```python
from build123d import *

# Parameters (mm, degrees)
SKETCH1_R           = 11.1125
BOSS_EXTRUDE1_DEPTH = 23.8125


with BuildPart() as part:
    # Sketch1 → Boss-Extrude1 (new body)
    with BuildSketch(Plane.XY):
        with BuildLine():
            Line((-19.45060256, -8.998474127), (-11.749724448, -25.644265115))
            Line((-11.749724448, -25.644265115), (12.863242985, -25.644265115))
            Line((12.863242985, -25.644265115), (19.45060256, -8.998474127))
            ThreePointArc((19.45060256, -8.998474127), (21.400108774, 1.154911696), (18.369201048, 11.039516721))
            Line((18.369201048, 11.039516721), (31.970540917, 23.950858732))
            Line((31.970540917, 23.950858732), (25.535140583, 31.951663088))
            Line((25.535140583, 31.951663088), (11.153892049, 18.299977287))
            ThreePointArc((11.153892049, 18.299977287), (-14.265700604, 15.993381845), (-19.45060256, -8.998474127))
        make_face()
        Circle(SKETCH1_R, mode=Mode.SUBTRACT)
    extrude(amount=BOSS_EXTRUDE1_DEPTH)


solid = part.part
```
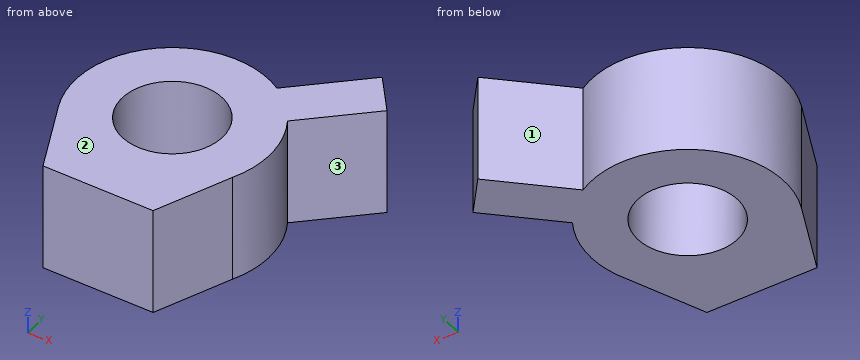
Input: part model. Units: mm. Frame: model coordinates. Face numbers are marked on the shaded views. A direction names the side the tool comes from. Round coordinates to 2 decimals unless told otherwise and drop trailing zeros. Loops run counter-clockwise (first coordinate to the right, second up) from the corner with the lowest first, then second, coordinate; pieces in that order, holes last.
1) Section query A-A on x = 0. Return the cut outline in (y, z), plus the area to 3 significant figures.
Ans:
outline: (-25.64, 0) - (-11.11, 0) - (-11.11, 23.81) - (-25.64, 23.81) - close; (11.11, 0) - (21.43, 0) - (21.43, 23.81) - (11.11, 23.81) - close
area: 592 mm2
2) Set-up query: the marked faces 1, 2 and 3. Return all of +Z, -Z, +X, -X, +Y, -Y with unobstructed straight access to the full face (end or side cutting, diameter ignored); none if empty.
Ans:
face 1: +Z, -Z, +Y
face 2: +Z, +X, -X, +Y, -Y
face 3: +Z, -Z, +X
3) Material intervals for line 1 (Y direction, x = 0, z = 15); line 2 (X direction, y = -3, z = 21.5); line 3 (Y direction, x = 4.5, z = 22), sorted ascending.
Ans:
line 1: y = -25.64 to -11.11, 11.11 to 21.43
line 2: x = -21.22 to -10.7, 10.7 to 21.22
line 3: y = -25.64 to -10.16, 10.16 to 20.95
4) Pin query (flat end, axial travel): pin 1 (1.5 mm diameter, centred on y = -9, z = 10, fed in from +X); pin 2 (10 mm diameter, centred on x = 4.5, y = 3.5, fed in from -Z); pin 3 (5 mm diameter, centred on x = -7.5, z = 12.5, fed in from +Y); pin 4 (1 mm diameter, centred on y = -15, z = 18, fed in from +X). Return the tip coordinate at first contact, or that it passes through.
Ans:
pin 1: stops at x = 19.78
pin 2: passes through
pin 3: stops at y = 20.84
pin 4: stops at x = 17.27
5) Section query C-C on z = 14. Return the cut outline in (x, y) (1 decimal).
Ans:
outline: (-19.5, -9) - (-11.7, -25.6) - (12.9, -25.6) - (19.5, -9) arc R21.4 ccw to (18.4, 11) - (32, 24) - (25.5, 32) - (11.2, 18.3) arc R21.4 ccw to start; hole circle Ø22.2 at (0, 0)
6) Section query D-D on y = 13.5. Return the cut outline in (x, z), plus the area to 3 significant figures.
Ans:
outline: (-16.64, 0) - (20.96, 0) - (20.96, 23.81) - (-16.64, 23.81) - close
area: 895 mm2
7) Section query B-B on y = 0. Return the cut outline in (x, z).
Ans:
outline: (-21.43, 0) - (-11.11, 0) - (-11.11, 23.81) - (-21.43, 23.81) - close; (11.11, 0) - (21.43, 0) - (21.43, 23.81) - (11.11, 23.81) - close
